Build history of the part. All positions in model axes, mm. A direction names the side the tool comes from. Round coordinates to 2 decimals unless told otherwise and drop trailing zeros. Write each loop counter-clockwise with the first axis right and the second up, starting at its lowest first coordinate (ties: lowest second). Pieces come first, ordered by that corner, then holes.
Autodesk Inventor part; units mm, degrees
ref_plane "YZ Plane" through (0, 0, 0) normal (1, 0, 0) x (0, 1, 0)
ref_plane "XZ Plane" through (0, 0, 0) normal (0, 1, 0) x (-1, 0, 0)
ref_plane "XY Plane" through (0, 0, 0) normal (0, 0, 1) x (1, 0, 0)
sketch "Esquisse1" plane through (0, 0, 0) normal (0, 0, 1) x (1, 0, 0)
  line L0 (22.5, 29) -> (-22.5, 29)
  line L1 (-26, 25.5) -> (-26, -25.5)
  line L2 (-22.5, -29) -> (22.5, -29)
  line L3 (26, -25.5) -> (26, 25.5)
  line L4 (26, 29) -> (-26, -29) construction
  line L5 (-26, 29) -> (26, -29) construction
  line L6 (-19, 6.5) -> (-19, 6.5)
  line L7 (-15.5, 3) -> (-15.5, -12)
  line L8 (-19, -15.5) -> (-19, -15.5)
  line L9 (-22.5, -12) -> (-22.5, 3)
  line L10 (-22.5, 6.5) -> (-15.5, -15.5) construction
  line L11 (-15.5, 6.5) -> (-22.5, -15.5) construction
  circle A0 centre (-19, 13) radius 3.5
  arc A1 (-22.5, -12) -> (-19, -15.5) centre (-19, -12) ccw
  arc A2 (-19, -15.5) -> (-15.5, -12) centre (-19, -12) ccw
  arc A3 (-19, 6.5) -> (-22.5, 3) centre (-19, 3) ccw
  arc A4 (-15.5, 3) -> (-19, 6.5) centre (-19, 3) ccw
  line L12 (0, 45.9017) -> (0, -37.4412)
  line L13 (15.5, 3) -> (15.5, -12)
  line L14 (22.5, -12) -> (22.5, 3)
  circle A5 centre (19, 13) radius 3.5
  arc A6 (19, -15.5) -> (22.5, -12) centre (19, -12) ccw
  arc A7 (15.5, -12) -> (19, -15.5) centre (19, -12) ccw
  arc A8 (22.5, 3) -> (19, 6.5) centre (19, 3) ccw
  arc A9 (19, 6.5) -> (15.5, 3) centre (19, 3) ccw
  arc A10 (-26, -25.5) -> (-22.5, -29) centre (-22.5, -25.5) ccw
  arc A11 (-22.5, 29) -> (-26, 25.5) centre (-22.5, 25.5) ccw
  arc A12 (26, 25.5) -> (22.5, 29) centre (22.5, 25.5) ccw
  arc A13 (22.5, -29) -> (26, -25.5) centre (22.5, -25.5) ccw
  point P0 (0, 0)
  point P1 (-19, -4.5)
  point P2 (19, -15.5)
  point P3 (19, 6.5)
  point P4 (-19, 6.5)
  point P5 (-19, -15.5)
  dimension "d0" = 52
  dimension "d1" = 58
  dimension "d2" = 7
  dimension "d5" = 3.5
  dimension "d6" = 7
  dimension "d7" = 42
  dimension "d8" = 3.5
  dimension "d9" = 15
  dimension "d10" = 17
  dimension "d12" = 0
  dimension "d13" = 3.5
extrude "Extrusion1" add sketch "Esquisse1" against normal blind 27
sketch "Esquisse2" plane through (0, 0, 0) normal (0, 0, 1) x (1, 0, 0)
  line L0 (-22.5, -29) -> (22.5, -29)
  circle A0 centre (19, 13) radius 3.5
  line L1 (19, 13) -> (19, -23)
  circle A1 centre (-19, 13) radius 3.5
  line L2 (-19, 13) -> (-19, 23)
  line L3 (22.5, 29) -> (-22.5, 29)
  point P0 (0, 0)
  dimension "d23" = 6
  dimension "d25" = 6
hole "Perçage1" at (19, -23, 0) at (-19, 23, 0) direction (0, 0, -1) diameter 4.134 depth 14.2 counterbore diameter 9 counterbore depth 3
sketch "Esquisse3" plane through (-22.5, 29, 0) normal (0, 1, 0) x (1, 0, 0)
  line L0 (45, 0) -> (0, 0)
  line L1 (45, 0) -> (45, 27)
  line L2 (0, 27) -> (45, 27)
  line L3 (0, 0) -> (0, 27)
  line L4 (32.5, 3.5) -> (12.5, 3.5)
  line L5 (12.5, 3.5) -> (12.5, 23.5)
  line L6 (12.5, 23.5) -> (32.5, 23.5)
  line L7 (32.5, 23.5) -> (32.5, 3.5)
  line L8 (32.5, 3.5) -> (12.5, 23.5) construction
  line L9 (12.5, 3.5) -> (32.5, 23.5) construction
  point P0 (22.5, 0)
  point P1 (22.5, 13.5)
  dimension "d26" = 20
  dimension "d27" = 20
extrude "Extrusion2" cut sketch "Esquisse3" against normal blind 50 contours L4 L5 L6 L7
properties part number "SupportTendeur"
1) Mould opens along Y. For faces 5 (the flat face through (19, -23, -14.2)), 6 (the flat face through (0, -21, -14)), 7 (the flat face through (-15.5, -4, -13)), 8 (the flat face through (0, 0, -27)) say: released by +Y, released by -Y, zero draft, split by the parting line, or undercut.
Results:
face 5: undercut
face 6: released by +Y
face 7: undercut
face 8: zero draft
2) Pin check, flat tips, straight feed: pin 1 Ø6 at (x, z) = (0.5, -18) entering from +Y; pin 2 Ø8 at (x, y) = (19, -23) entering from +Z; pin 3 Ø1 at (x, y) = (16.5, -7.5) entering from +Z; pin 4 Ø2 at (x, y) = (-19.5, 23.5) entering from +Z. Stop position of each tip, or through.
Results:
pin 1: stops at y = -21
pin 2: stops at z = -3
pin 3: passes through
pin 4: stops at z = -14.2
3) Slice it at C-C (z = -24.75). Write the cut outline in (x, y).
Results:
outline: (-26, -25.5) arc R3.5 ccw to (-22.5, -29) - (22.5, -29) arc R3.5 ccw to (26, -25.5) - (26, 25.5) arc R3.5 ccw to (22.5, 29) - (-22.5, 29) arc R3.5 ccw to (-26, 25.5) - close; hole (-22.5, -12) arc R3.5 ccw to (-15.5, -12) - (-15.5, 3) arc R3.5 ccw to (-22.5, 3) - close; hole circle Ø7 at (-19, 13); hole (15.5, -12) arc R3.5 ccw to (22.5, -12) - (22.5, 3) arc R3.5 ccw to (15.5, 3) - close; hole circle Ø7 at (19, 13)
4) Wall check: L1, parallel to Y at x = -19, z = -0.85; L2, parallel to Y at x = 19, z = -1.3; L3, parallel to X at y = -8.5, z = -10. Give the ranges that are in metal, low to high.
Results:
L1: y = -29 to -15.5, 6.5 to 9.5, 16.5 to 18.5, 27.5 to 29
L2: y = -29 to -27.5, -18.5 to -15.5, 6.5 to 9.5, 16.5 to 29
L3: x = -26 to -22.5, -15.5 to -10, 10 to 15.5, 22.5 to 26
5) Slice it at B-B (x = 9). Write the cut outline in (y, z), plus the area to 3 significant figures.
Results:
outline: (-29, -27) - (29, -27) - (29, -23.5) - (-21, -23.5) - (-21, -3.5) - (29, -3.5) - (29, 0) - (-29, 0) - close
area: 566 mm2
6) Slice it at D-D (y = 23). Write the cut outline in (x, z), plus the area to 3 significant figures.
Results:
outline: (-26, -27) - (26, -27) - (26, 0) - (-14.5, 0) - (-14.5, -3) - (-16.93, -3) - (-16.93, -14.2) - (-21.07, -14.2) - (-21.07, -3) - (-23.5, -3) - (-23.5, 0) - (-26, 0) - close; hole (-10, -23.5) - (10, -23.5) - (10, -3.5) - (-10, -3.5) - close
area: 931 mm2
7) Which spindle directions (+Z, -Z, +X, -X, +Y, -Y) get a long thin tool onto all of the face, cutting with end or side? Do faces 1 (the flat face through (21, -24, -3)), 2 (the flat face through (0, 4, -23.5)), 3 (the cylindrical face through (-25, -27.95, -13.31)), 4 (the flat face through (15.5, -4, -13)). Say none if no direction does.
Results:
face 1: +Z
face 2: +Y
face 3: +Z, -Z, -X, -Y
face 4: +Z, -Z
8) Slice it at A-A (y = 13). Write the cut outline in (x, z), plus the area to 3 significant figures.
Results:
outline: (-26, -27) - (-22.5, -27) - (-22.5, 0) - (-26, 0) - close; (-15.5, -27) - (15.5, -27) - (15.5, 0) - (-15.5, 0) - close; (22.5, -27) - (26, -27) - (26, 0) - (22.5, 0) - close; hole (-10, -23.5) - (10, -23.5) - (10, -3.5) - (-10, -3.5) - close
area: 626 mm2
